Input: part model. Units: mm. Frame: model coordinates. A direction names the side the tool comes from. Coordinates: 2 decimals unless noted, no trailing zeros. Write each loop counter-clockwise with the first axis right and the second up, starting at its lowest first coordinate (ties: lowest second). Pieces come first, ordered by that corner, then holes.
1) Section query D-D (z = -2134). Output: boundary loops of the cut face in (x, y), then the cut area to 3 significant figures.
2) Set-up query: faces 1 (the flat face through (142, 2, -1186)), 2 (the flat face through (1, -119, -2405)). Return all of +Z, -Z, +X, -X, +Y, -Y with unobstructed straight access to the full face (end or side cutting, diameter ignored); none if empty.
3) Line query: L1, parallel to Z at x = -147.75, y = -96.5; L2, parallel to X at y = 53.5, z = -818.5; L3, parallel to Y at x = 1.5, z = -412.5. Output: solid intervals per line, ascending.
4) Section query C-C (y = 0). Output: boundary loops of the cut face in (x, z).
5) Pin query (flat end, axial travel): pin 1 Ø2.5 at (y, z) = (-119.5, -2040.5) entering from -X; pin 2 Ø2.5 at (y, z) = (-120.5, -2046.5) entering from +X; pin 3 Ø1.5 at (x, z) = (11, -2085) entering from +Y. Return the tip coordinate at first contact, or that it passes through.
6) Draft query along Z for faces 3 (the cylindrical face through (-145.94, -9.76, -2177.93)), 4 (the flat face through (0.7, 121.142, -2047.611)), 5 (the flat face through (-2, 117, -1014)). Return one class per face: pulls with the +Z half, pulls with the -Z half, needs draft (parallel to the pull), parting line crosses it, or undercut.
7) Section query A-A (x = -1.5). Output: boundary loops of the cut face in (y, z), then the cut area to 3 significant figures.
8) Section query B-B (z = -219.5). Output: boundary loops of the cut face in (x, y).
from build123d import *

# Parameters (mm, degrees)
EXTRUDE_1_DEPTH     = 2405
SKETCH_2_R          = 8
SKETCH_2_R_2        = 45
CUT_EXTRUDE_1_DEPTH = 2427.860111337
CUT_EXTRUDE_2_REACH = 2424.607
SKETCH_3_W          = 70
SKETCH_3_H          = 90


with BuildPart() as part:
    # 草图1 → 凸台-拉伸1 (new body)
    with BuildSketch(Plane.XY):
        with BuildLine():
            Line((-134, 125), (134, 125))
            ThreePointArc((134, 125), (145.313708499, 120.313708499), (150, 109))
            Line((150, 109), (150, -109))
            ThreePointArc((150, -109), (145.313708499, -120.313708499), (134, -125))
            Line((134, -125), (-134, -125))
            ThreePointArc((-134, -125), (-145.313708499, -120.313708499), (-150, -109))
            Line((-150, -109), (-150, 109))
            ThreePointArc((-150, 109), (-145.313708499, 120.313708499), (-134, 125))
        make_face()
        with BuildLine():
            Line((-134, 117), (134, 117))
            ThreePointArc((134, 117), (139.656854249, 114.656854249), (142, 109))
            Line((142, 109), (142, -109))
            ThreePointArc((142, -109), (139.656854249, -114.656854249), (134, -117))
            Line((134, -117), (-134, -117))
            ThreePointArc((-134, -117), (-139.656854249, -114.656854249), (-142, -109))
            Line((-142, -109), (-142, 109))
            ThreePointArc((-142, 109), (-139.656854249, 114.656854249), (-134, 117))
        make_face(mode=Mode.SUBTRACT)
    extrude(amount=-EXTRUDE_1_DEPTH)

    # 草图2 → 切除-拉伸1 (cut, through all)
    with BuildSketch(Plane(origin=(150, 0, 0), x_dir=(0, 0, -1), z_dir=(1, 0, 0))):
        with Locations(Location((35, 96.5, 0), (0, 0, 90))):
            Circle(SKETCH_2_R)
        with Locations(Location((175, 96.5, 0), (0, 0, 90))):
            Circle(SKETCH_2_R)
        with Locations(Location((315, 96.5, 0), (0, 0, 90))):
            Circle(SKETCH_2_R)
        with Locations(Location((2134, 0, 0), (0, 0, 90))):
            Circle(SKETCH_2_R_2)
        with Locations(Location((315, -96.5, 0), (0, 0, 180))):
            Circle(SKETCH_2_R)
        with Locations(Location((175, -96.5, 0), (0, 0, 180))):
            Circle(SKETCH_2_R)
        with Locations(Location((35, -96.5, 0), (0, 0, 180))):
            Circle(SKETCH_2_R)
        Polygon((2405, -60), (2040, 125), (2405, 125), align=None)
    extrude(amount=-CUT_EXTRUDE_1_DEPTH, mode=Mode.SUBTRACT)

    # 草图3 → 切除-拉伸2 (cut, up to next)
    with BuildSketch(Plane.XZ.offset(125), mode=Mode.PRIVATE) as cut_extrude_2_sk1:
        with Locations((0, -2025.5)):
            Rectangle(SKETCH_3_W, SKETCH_3_H)
    cut_extrude_2_tool1 = extrude(cut_extrude_2_sk1.sketch, amount=-CUT_EXTRUDE_2_REACH, mode=Mode.PRIVATE) & part.part
    add(cut_extrude_2_tool1.solids().sort_by_distance((0, -125, -2025.5))[0], mode=Mode.SUBTRACT)


solid = part.part
Answer:
1. outline: (-150, -109) arc R16 ccw to (-134, -125) - (134, -125) arc R16 ccw to (150, -109) - (150, -45) - (142, -45) - (142, -109) arc R8 cw to (134, -117) - (-134, -117) arc R8 cw to (-142, -109) - (-142, -45) - (-150, -45) - close; (-150, 45) - (-142, 45) - (-142, 77.36) - (-150, 77.36) - close; (142, 45) - (150, 45) - (150, 77.36) - (142, 77.36) - close
1. area: 3,990 mm2
2. face 1: +Z, -Z
2. face 2: -Z, +X, -X, +Y, -Y
3. L1: z = -2405 to -323, -307 to -183, -167 to -43, -27 to 0
3. L2: x = -150 to -142, 142 to 150
3. L3: y = -125 to -117, 117 to 125
4. outline: (-150, -2286.62) - (-142, -2286.62) - (-142, -2179) - (-150, -2179) - close; (-150, -2089) - (-142, -2089) - (-142, 0) - (-150, 0) - close; (142, -2286.62) - (150, -2286.62) - (150, -2179) - (142, -2179) - close; (142, -2089) - (150, -2089) - (150, 0) - (142, 0) - close
5. pin 1: stops at x = -147.06
5. pin 2: stops at x = 146.29
5. pin 3: stops at y = -117
6. face 3: undercut
6. face 4: pulls with the -Z half
6. face 5: needs draft
7. outline: (-125, -2405) - (-117, -2405) - (-117, -2070.5) - (-125, -2070.5) - close; (-125, -1980.5) - (-117, -1980.5) - (-117, 0) - (-125, 0) - close; (117, -2055.78) - (125, -2040) - (125, 0) - (117, 0) - close
7. area: 34,900 mm2
8. outline: (-150, -109) arc R16 ccw to (-134, -125) - (134, -125) arc R16 ccw to (150, -109) - (150, 109) arc R16 ccw to (134, 125) - (-134, 125) arc R16 ccw to (-150, 109) - close; hole (-142, -109) arc R8 ccw to (-134, -117) - (134, -117) arc R8 ccw to (142, -109) - (142, 109) arc R8 ccw to (134, 117) - (-134, 117) arc R8 ccw to (-142, 109) - close
